Verification items for the finished model (mm, model axes). A direction names the side the tool comes from. Round coordinates to 2 decimals unless told otherwise and drop trailing zeros. Write each loop counter-clockwise with the first axis right and the second up, starting at its lowest first coordinate (ties: lowest second). Pieces come first, ordered by that corner, then holes. Notation, with made-up numbers: (57.25, 63.25) - (107.25, 63.25) arc R11 cw to (107.25, 67.25) - close; hole circle Ø4 at (6.25, -10.75). An arc over 180 degrees is marked (long way). Answer as a JSON object with one key per item and string values.
```python
from build123d import *

# Parameters (mm, degrees)
SKETCH2_R               = 9.525
BOSS_EXTRUDE1_DEPTH     = 10
SKETCH3_R               = 1.5
CUT_EXTRUDE1_DEPTH      = 15.2875
CUT_EXTRUDE1_DEPTH_BACK = 5.7625


with BuildPart() as part:
    # Sketch2 → Boss-Extrude1 (new body)
    with BuildSketch(Plane.XY):
        Circle(SKETCH2_R)
        Polygon((5.499261314, 0), (2.749630657, 4.7625), (-2.749630657, 4.7625), (-5.499261314, 0), (-2.749630657, -4.7625), (2.749630657, -4.7625), align=None, mode=Mode.SUBTRACT)
    extrude(amount=BOSS_EXTRUDE1_DEPTH)

    # Sketch3 → Cut-Extrude1 (cut, two sides)
    with BuildSketch(Plane(origin=(0, -4.7625, 0), x_dir=(1, 0, 0), z_dir=(0, 1, 0))) as cut_extrude1_sk:
        with Locations((0, -5)):
            Circle(SKETCH3_R)
    extrude(amount=CUT_EXTRUDE1_DEPTH, mode=Mode.SUBTRACT)
    extrude(cut_extrude1_sk.sketch, amount=-CUT_EXTRUDE1_DEPTH_BACK, mode=Mode.SUBTRACT)


solid = part.part
```
1. Mould release check, pull along Z, two halves, no side actions. Record for faces 1 (the face through (-0.195, 7.112, 3.513)), 2 (the face through (-4.4, 2.3, 0)), 3 (the face through (-0.195, -7.112, 3.513)), 4 (the face through (-1.2, 4.762, 3.8)): released by +Z, released by -Z, zero draft, split by the parting line, or undercut.
Completed:
{"face 1": "undercut", "face 2": "released by -Z", "face 3": "undercut", "face 4": "zero draft"}
2. Cross-section at A-A (x = 0). Record the boundary of the cut face in (y, z) (1 decimal).
Completed:
{"outline": "(-9.5, 0) - (-4.8, 0) - (-4.8, 3.5) - (-9.5, 3.5) - close; (-9.5, 6.5) - (-4.8, 6.5) - (-4.8, 10) - (-9.5, 10) - close; (4.8, 0) - (9.5, 0) - (9.5, 3.5) - (4.8, 3.5) - close; (4.8, 6.5) - (9.5, 6.5) - (9.5, 10) - (4.8, 10) - close"}
3. Access from +Z, -Z, +X, -X, +Y, -Y to the whole of each face (thin tool, end or side, straight path). Record for faces 5 (the face through (1.2, -4.762, 3.8)), 6 (the face through (-4.4, 2.3, 10)).
Completed:
{"face 5": "+Z, -Z", "face 6": "+Z, +X, -X, +Y, -Y"}
4. Cross-section at C-C (y = -3.5). Record the boundary of the cut face in (x, z).
Completed:
{"outline": "(-8.86, 0) - (-3.48, 0) - (-3.48, 10) - (-8.86, 10) - close; (3.48, 0) - (8.86, 0) - (8.86, 10) - (3.48, 10) - close"}
5. Material ranges on probe 1 along Z at (x, y) = (0, 8.2); probe 2 along X at (y, z) = (8.45, 5); probe 3 along Y at (x, z) = (-4.75, 4.25), recorded low to high. Write a range as from..to.
Completed:
{"probe 1": "z = 0..3.5, 6.5..10", "probe 2": "x = -4.4..-1.5, 1.5..4.4", "probe 3": "y = -8.26..-1.3, 1.3..8.26"}
6. Go/stop test with flat-tipped pins: pin 1 (1.5 mm diameter, centred on y = -7, z = 7, fed in from -X); pin 2 (6 mm diameter, centred on y = -7, z = 2, fed in from +X). Record where each tip stops, or that it passes through.
Completed:
{"pin 1": "stops at x = -7.19", "pin 2": "stops at x = 8.64"}
7. Cross-section at D-D (x = 2). Record the boundary of the cut face in (y, z), plus the area to 3 significant figures.
Completed:
{"outline": "(-9.31, 0) - (-4.76, 0) - (-4.76, 10) - (-9.31, 10) - close; (4.76, 0) - (9.31, 0) - (9.31, 10) - (4.76, 10) - close", "area": "91.0 mm^2"}
